from build123d import *

# Parameters (mm, degrees)
ESQUISSE1_R        = 1
BOSS_EXTRU_1_DEPTH = 5


with BuildPart() as part:
    # Esquisse1 → Boss.-Extru.1 (new body)
    with BuildSketch(Plane.XY):
        Polygon((0, 0), (0, 212), (20, 212), (20, 206), (85, 206), (85, 212), (115, 212), (115, 206), (180, 206), (180, 212), (200, 212), (200, 0), (180, 0), (180, 6), (115, 6), (115, 0), (85, 0), (85, 6), (20, 6), (20, 0), align=None)
        with Locations((170, 36)):
            Circle(ESQUISSE1_R, mode=Mode.SUBTRACT)
        with Locations((96.8, 36)):
            Circle(ESQUISSE1_R, mode=Mode.SUBTRACT)
        with Locations((96.8, 130.2)):
            Circle(ESQUISSE1_R, mode=Mode.SUBTRACT)
        with Locations((170, 130.2)):
            Circle(ESQUISSE1_R, mode=Mode.SUBTRACT)
    extrude(amount=BOSS_EXTRU_1_DEPTH)


solid = part.part
Source: CAD feature listing. Evaluate the final solid. Frame: model axes, mm. A direction names the side the tool comes from. Round coordinates to 2 decimals unless told otherwise and drop trailing zeros. Loops run counter-clockwise (first coordinate to the right, second up) from the corner with the lowest first, then second, coordinate; pieces in that order, holes last. Notation, with made-up numbers: (23, 56) -> (76, 56) arc R24 cw to (76, 83) -> close; hole circle Ø4 at (63, 57.25). An arc over 180 degrees is marked (long way). Answer as a JSON object with one key per item and string values. Group by question number.
Q1. Section query B-B (x = 78.5). Output: boundary loops of the cut face in (y, z).
Q2. Ray query, line 1 (Y direction, x = 170, z = 2.4); line 2 (Y direction, x = 96.8, z = 3.05); line 3 (X direction, y = 130.2, z = 3.2). Return the intervals inside material, ascending. Write a range as from..to.
Q3. Contact query for flat-ended pins moving along their axis: P1, Ø1.5, axis at x = 60.5, z = 1.5, coming from the +Y side; P2, Ø1, axis at x = 116.5, z = 3, coming from the -Y side. Output: stop coordinate, or through.
Q4. Section query A-A (z = 4.1). Output: boundary loops of the cut face in (x, y), plus the area to 3 significant figures.
Q5. Access query for faces 1 (the flat face through (10, 212, 2)), 2 (the flat face through (180, 3, 2)), 3 (the flat face through (20, 209, 2)). Directions: +Z, -Z, +X, -X, +Y, -Y. A direction counts if a zero-diameter tool reaches every point of the face in a straight line with its end or side. Return the directions, or none.
Completed:
{
 "1": {"outline": "(6, 0) -> (206, 0) -> (206, 5) -> (6, 5) -> close"},
 "2": {"line 1": "6..35, 37..129.2, 131.2..206", "line 2": "0..35, 37..129.2, 131.2..212", "line 3": "0..95.8, 97.8..169, 171..200"},
 "3": {"P1": "y = 206", "P2": "y = 6"},
 "4": {"outline": "(0, 0) -> (20, 0) -> (20, 6) -> (85, 6) -> (85, 0) -> (115, 0) -> (115, 6) -> (180, 6) -> (180, 0) -> (200, 0) -> (200, 212) -> (180, 212) -> (180, 206) -> (115, 206) -> (115, 212) -> (85, 212) -> (85, 206) -> (20, 206) -> (20, 212) -> (0, 212) -> close; hole circle Ø2 at (96.8, 36); hole circle Ø2 at (96.8, 130.2); hole circle Ø2 at (170, 36); hole circle Ø2 at (170, 130.2)", "area": "40,800 mm²"},
 "5": {"face 1": "+Z, -Z, +X, -X, +Y", "face 2": "+Z, -Z, -Y", "face 3": "+Z, -Z, +Y"}
}
